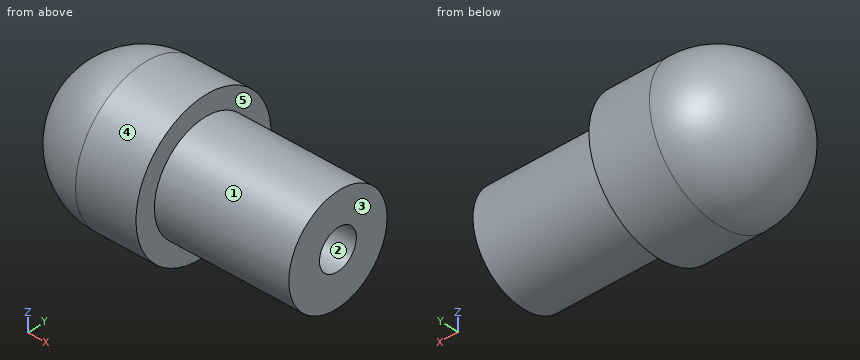
```python
from build123d import *

# Parameters (mm, degrees)
SKETCH4_R          = 1.5
CUT_EXTRUDE1_DEPTH = 14.5


with BuildPart() as part:
    # Sketch3 → Revolve1 (revolve)
    with BuildSketch(Plane.XY, mode=Mode.PRIVATE) as revolve1_sk:
        with BuildLine():
            Line((5.5, 5.5), (10, 5.5))
            Line((10, 5.5), (10, 4))
            Line((10, 4), (20, 4))
            Line((20, 4), (20, 0))
            Line((20, 0), (0, 0))
            ThreePointArc((0, 0), (1.610912703, 3.889087297), (5.5, 5.5))
        make_face()
    revolve(revolve1_sk.sketch.rotate(Axis((0, 0, 0), (-1, 0, 0)), 90), axis=Axis((0, 0, 0), (-1, 0, 0)))

    # Sketch4 → Cut-Extrude1 (cut)
    with BuildSketch(Plane(origin=(20, 0, 0), x_dir=(0, 0, -1), z_dir=(1, 0, 0))):
        Circle(SKETCH4_R)
    extrude(amount=-CUT_EXTRUDE1_DEPTH, mode=Mode.SUBTRACT)


solid = part.part
```
Here's how the part is built. I have some questions about the finished solid (model axes, mm). Face numbers are marked on the shaded views. A direction names the side the tool comes from. Coordinates: 2 decimals unless noted, no trailing zeros. Loops run counter-clockwise (first coordinate to the right, second up) from the corner with the lowest first, then second, coordinate; pieces in that order, holes last. Notation, with made-up numbers: (17.5, 28) - (49.5, 28) arc R9 ccw to (49.5, 45) - close; hole circle Ø5 at (8.5, 37.25). An arc over 180 degrees is marked (long way). Answer as CSV lines item,"result".
Q1. If we section it at A-A, the plane z = 0: Write out the boundary of the cut face in (x, y).
Response:
outline,"(5.5, -5.5) - (10, -5.5) - (10, -4) - (20, -4) - (20, -1.5) - (5.5, -1.5) - (5.5, 1.5) - (20, 1.5) - (20, 4) - (10, 4) - (10, 5.5) - (5.5, 5.5) arc R5.5 ccw to start"
Q2. We'd pull the mould along Y, two halves only. Please class the marked faces 1, 2 and 3: pulls with the +Y half, pulls with the -Y half, needs draft (parallel to the pull), parting line crosses it, or undercut.
Response:
face 1,"parting line crosses it"
face 2,"undercut"
face 3,"needs draft"
Q3. For pin 1 (5 mm diameter, centred on x = 13.5, y = 0.5, fed in from -Z); pin 2 (6 mm diameter, centred on y = -2.5, z = -1.5, fed in from -X); pin 3 (2 mm diameter, centred on x = 3, y = -1.5, fed in from +Z); pin 4 (5 mm diameter, centred on x = 17, y = 3.5, fed in from -Z), each with a flat end and sliding along its axis, tell me the tip position at first contact or that it passes through.
Response:
pin 1,"z = -4"
pin 2,"x = 0"
pin 3,"z = 5.16"
pin 4,"z = -3.87"
Q4. For the marked faces 4 and 5, which set-ups out of +Z, -Z, +X, -X, +Y, -Y let a thin tool reach every point of the face, with its end or its side?
Response:
face 4,"+X, -X"
face 5,"+X"
Q5. If we section it at D-D, the plane x = 18.25: Write out the boundary of the cut face in (y, z).
Response:
outline,"circle Ø8 at (0, 0); hole circle Ø3 at (0, 0)"
Q6. If we section it at C-C, the plane x = 9.5: Write out the boundary of the cut face in (y, z).
Response:
outline,"circle Ø11 at (0, 0); hole circle Ø3 at (0, 0)"
Q7. If I drill on L1, parallel to Y at x = 12, z = 0; L2, parallel to Z at x = 11.75, y = -1.25; L3, parallel to Y at x = 17.5, z = 0.5, over which ranges is the centre line in solid material (lowest first)? Write a range as [from, to].
Response:
L1,"[-4, -1.5], [1.5, 4]"
L2,"[-3.8, -0.83], [0.83, 3.8]"
L3,"[-3.97, -1.41], [1.41, 3.97]"
